```python
from build123d import *

# Parameters (mm, degrees)
SKETCH_R         = 2.5
PAD_DEPTH        = 2.4
POCKET_START     = -3
SKETCH001_W      = 171.051082
SKETCH001_H      = 1.4
POCKET_DEPTH     = 4
CHAMFER001_SIZE2 = 3
CHAMFER001_SIZE  = 0.7
CHAMFER002_SIZE2 = 3
CHAMFER002_SIZE  = 0.7
FILLET001_R      = 2
CHAMFER003_SIZE  = 0.5
CHAMFER004_SIZE  = 0.7


with BuildPart() as part:
    # Sketch (on Origin) → Pad (new body)
    with BuildSketch(Plane.XY):
        Polygon((-88.571429, 0), (0, 0), (0, -150), (-35, -150), align=None)
        with Locations((-30, -10)):
            Circle(SKETCH_R, mode=Mode.SUBTRACT)
    extrude(amount=PAD_DEPTH)

    # Sketch001 (on Face4 of Pad) → Pocket (cut)
    with BuildSketch(Plane(origin=(-78.552036, -28.054299, 0), x_dir=(0.336336, -0.941742, 0), z_dir=(-0.941742, -0.336336, 0)).offset(POCKET_START)):
        with Locations((55.735746, 1.7)):
            Rectangle(SKETCH001_W, SKETCH001_H)
    extrude(amount=-POCKET_DEPTH, mode=Mode.SUBTRACT)

    # Chamfer001
    chamfer001_edges = [part.edges().sort_by_distance(p)[0] for p in [
        (0, -75, 2.4),
    ]]
    chamfer001_side = part.faces().sort_by_distance((0, -75, 1.2))[0]
    chamfer(chamfer001_edges, length=CHAMFER001_SIZE, length2=CHAMFER001_SIZE2, reference=chamfer001_side)

    # Chamfer002
    chamfer002_edges = [part.edges().sort_by_distance(p)[0] for p in [
        (0, -75, 0),
    ]]
    chamfer002_side = part.faces().sort_by_distance((0, -75, 0.85))[0]
    chamfer(chamfer002_edges, length=CHAMFER002_SIZE, length2=CHAMFER002_SIZE2, reference=chamfer002_side)

    # Fillet001
    fillet001_edges = [part.edges().sort_by_distance(p)[0] for p in [
        (-35, -150, 1.2),
        (-88.571429, 0, 1.2),
    ]]
    fillet(fillet001_edges, radius=FILLET001_R)

    # Chamfer003
    chamfer003_edges = [part.edges().sort_by_distance(p)[0] for p in [
        (-18.295281, -150, 0),
        (-61.545474, -75.672673, 2.4),
        (-42.069197, 0, 2.4),
        (-15.283483, -150, 2.4),
    ]]
    chamfer(chamfer003_edges, length=CHAMFER003_SIZE)

    # Chamfer004
    chamfer004_edges = [part.edges().sort_by_distance(p)[0] for p in [
        (-27.5, -10, 1.2),
        (-32.5, -10, 0),
        (-32.5, -10, 2.4),
    ]]
    chamfer(chamfer004_edges, length=CHAMFER004_SIZE)


solid = part.part
```
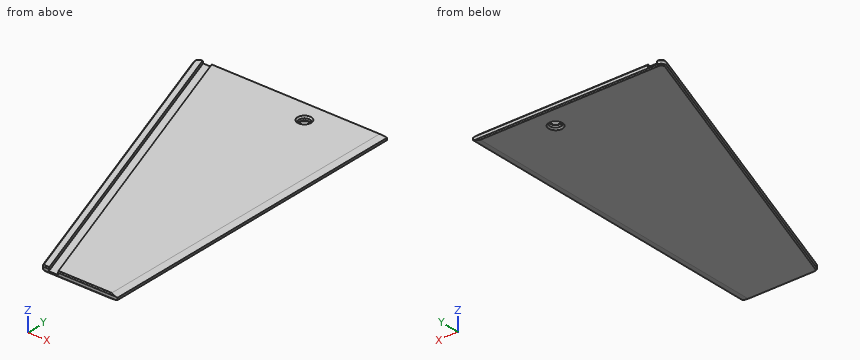
Design review of the part built by this model. Coordinates are the model's own, in mm. Give positions to 0.01 mm unless a question says otherwise; leave off trailing zeros. Write each loop counter-clockwise with the first axis right and the second up, starting at its lowest first coordinate (ties: lowest second). Pieces come first, ordered by that corner, then holes.
(1) Add section C-C (y = -58.5). Give the boundary of the cut face in (x, z).
Checked values:
outline: (-67.68, 0.5) - (-67.15, 0) - (-3, 0) - (0, 0.7) - (0, 1.7) - (-3, 2.4) - (-60.25, 2.4) - (-60.25, 1) - (-64.49, 1) - (-64.49, 2.4) - (-67.15, 2.4) - (-67.68, 1.9) - close
(2) Add section A-A (x = -30). Give the boundary of the cut face in (y, z).
Checked values:
outline: (-150, 0.5) - (-149.5, 0) - (-13.2, 0) - (-12.5, 0.7) - (-12.5, 1.7) - (-13.2, 2.4) - (-143.19, 2.4) - (-143.19, 1) - (-150, 1) - close; (-7.5, 0.7) - (-6.8, 0) - (-0.5, 0) - (0, 0.5) - (0, 1.9) - (-0.5, 2.4) - (-6.8, 2.4) - (-7.5, 1.7) - close
(3) Add section B-B (y = -10). Give the boundary of the cut face in (x, z).
Checked values:
outline: (-85, 0.5) - (-84.47, 0) - (-33.2, 0) - (-32.5, 0.7) - (-32.5, 1.7) - (-33.2, 2.4) - (-77.57, 2.4) - (-77.57, 1) - (-81.81, 1) - (-81.81, 2.4) - (-84.47, 2.4) - (-85, 1.9) - close; (-27.5, 0.7) - (-26.8, 0) - (-3, 0) - (0, 0.7) - (0, 1.7) - (-3, 2.4) - (-26.8, 2.4) - (-27.5, 1.7) - close
(4) Wall thickness on line 1 along Z through (x, y) = (-43, -127.5); line 2 along X through (y, z) = (-65.5, 1.2); line 3 along X through (y, z) = (-99, 1.5): over which ranges is each line inside the solid? List them lowest first.
Checked values:
line 1: z = 0.47 to 1.93
line 2: x = -65.18 to -61.99, -57.75 to 0
line 3: x = -53.21 to -50.03, -45.78 to 0
(5) Add section D-D (x = -77). Give the boundary of the cut face in (y, z).
Checked values:
outline: (-32.4, 0.5) - (-30.91, 0) - (-0.5, 0) - (0, 0.5) - (0, 1.9) - (-0.5, 2.4) - (-11.59, 2.4) - (-11.59, 1) - (-23.48, 1) - (-23.48, 2.4) - (-30.91, 2.4) - (-32.4, 1.9) - close
